```python
from build123d import *

# Parameters (mm, degrees)
F0_R     = 4.7625
F1_DEPTH = 152.908
F2_SIZE2 = 1.27
F2_SIZE  = 1.27
F3_R     = 3.175
F4_DEPTH = 24.892


with BuildPart() as f1:
    # F0 (on Front) → F1 (new body)
    with BuildSketch(Plane.XZ):
        Circle(F0_R)
    extrude(amount=F1_DEPTH)

    # F2
    f2_edges = [f1.edges().sort_by_distance(p)[0] for p in [
        (-4.7625, -152.908, 0),
        (-4.7625, 0, 0),
    ]]
    chamfer(f2_edges, length=F2_SIZE, length2=F2_SIZE2)

    # F3 (on face) → F4 (join)
    with BuildSketch(Plane(origin=(0, 0, 0), x_dir=(-1, 0, 0), z_dir=(0, 1, 0))):
        Circle(F3_R)
    extrude(amount=F4_DEPTH)


solid = f1.part
```
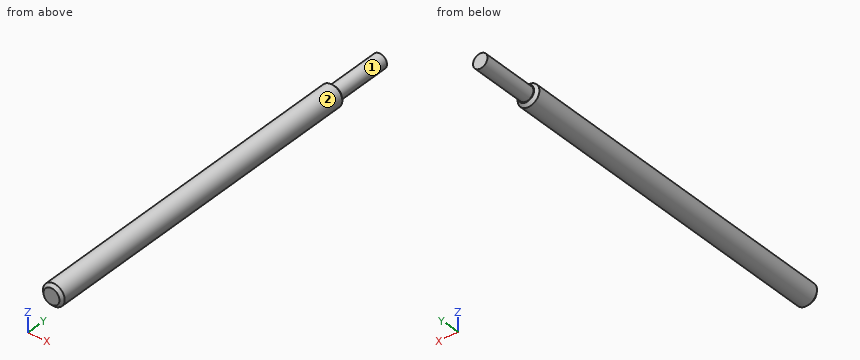
Input: part model. Units: mm. Frame: model coordinates. Face numbers are marked on the shaded views. A direction names the side the tool comes from. Give positions to 0.01 mm unless a question says otherwise; leave off trailing zeros. Order: outer loops, then holes, each group sorted by start corner. A loop starts at its lowest first (then second) coordinate and runs counter-clockwise, first axis right, second up. Notation, with made-up numbers: (-22.5, 85) - (35.5, 85) arc R29 cw to (35.5, 109) - close; hole circle Ø5 at (55, -24.5). An arc over 180 degrees is marked (long way). One line per item, written item: value.
1. Line query: probe 1 along Y at (x, z) = (-0.75, -3.25); probe 2 along X at (y, z) = (-20.5, -0.5); probe 3 along X at (y, z) = (-138.5, 3.25). Output: solid intervals per line, ascending.
Determined:
probe 1: -152.91 to 0
probe 2: -4.74 to 4.74
probe 3: -3.48 to 3.48
2. Pin query (flat end, axial travel): pin 1 Ø2 at (x, z) = (-3.5, -2.5) entering from +Y; pin 2 Ø5 at (y, z) = (4.5, 2) entering from -X (3 decimals); pin 3 Ø2 at (x, y) = (1, -77.5) entering from -Z; pin 4 Ø1 at (y, z) = (-14.5, 4) entering from +X. Return the tip coordinate at first contact, or that it passes through.
Determined:
pin 1: y = 0
pin 2: x = -3.175
pin 3: z = -4.76
pin 4: x = 3.23
3. Reachability of the marked faces 1 and 2 from +Z, -Z, +X, -X, +Y, -Y: full face, straight path, thin tool, end or side. Return the list, or none.
Determined:
face 1: +Y
face 2: +Y, -Y
4. Cut plane C-C, the plane y = -42. Output: boundary loops of the cut face in (x, z) (1 decimal).
Determined:
outline: circle Ø9.5 at (0, 0)
